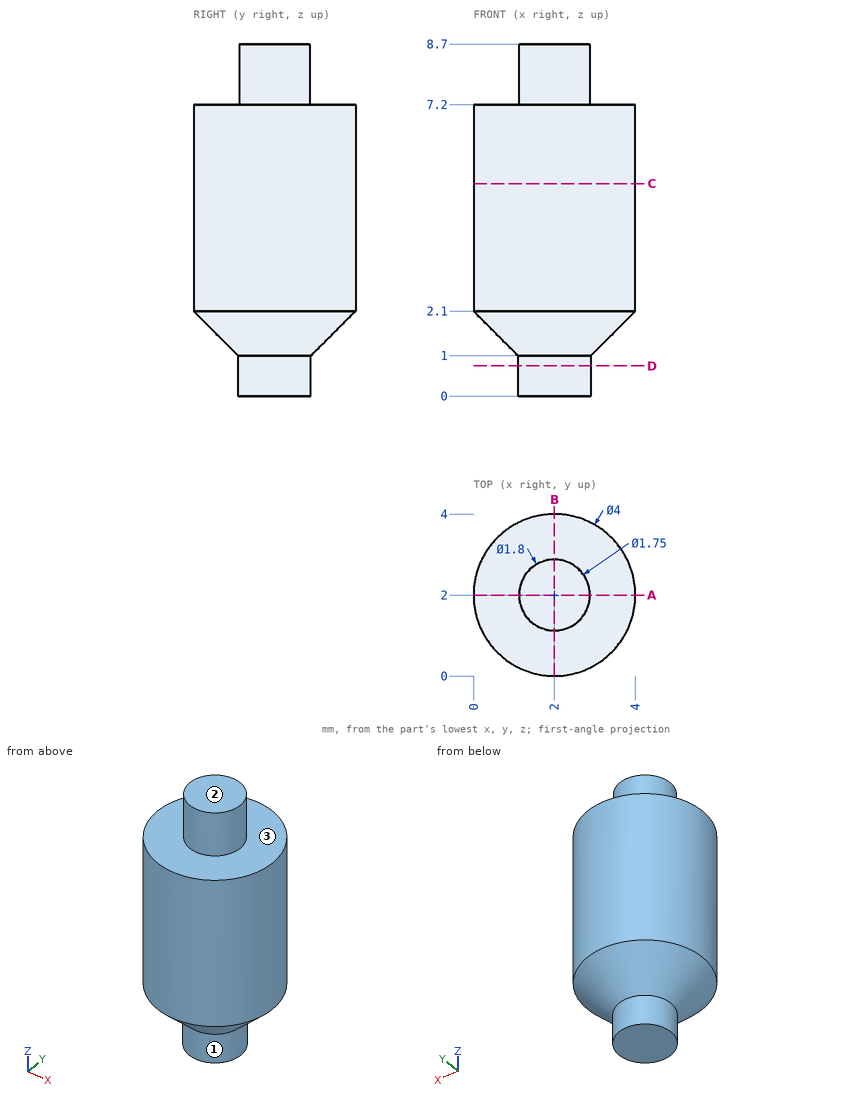
Here's the drawing with two shaded views (mm, measured from the low corner). I have some questions. A direction names the side the tool comes from. Give positions to 0.01 mm unless a question says otherwise; leave off trailing zeros. Loops run counter-clockwise (first coordinate to the right, second up) from the corner with the lowest first, then second, coordinate; pieces in that order, holes last. Notation, with made-up numbers: M 81.25,86.5 L 119.25,86.5 A15 ccw 119.25,113.5 Z; hole C 86,-17 d2. An arc over 180 degrees is marked long. One line per item, written item: value.
(1) Suppose I cut it at D-D on z = 0.75. List the corners of the cut face in (x, y) for me.
Returned:
outline: C 2,2 d1.8
(2) Will this pin go through, and if not, where does the flat tip stop? pin 1 (1.5 mm diameter, centred on x = 2, y = 3, fed in from +Z).
Returned:
pin 1: z = 8.7
(3) Suppose I cut it at C-C on z = 5.25. List the corners of the cut face in (x, y) for me.
Returned:
outline: C 2,2 d4
(4) Which directions (+Z, -Z, +X, -X, +Y, -Y) give clear straight access to the entire face, cutting with the end or side of a thin tool? Please do the marked faces 1, 2 and 3.
Returned:
face 1: -Z
face 2: +Z, +X, -X, +Y, -Y
face 3: +Z
(5) Suppose I cut it at A-A on y = 2. List the corners of the cut face in (x, z) for me (3 decimals).
Returned:
outline: M 0,2.1 L 1.1,1 L 1.1,0 L 2.9,0 L 2.9,1 L 4,2.1 L 4,7.2 L 2.875,7.2 L 2.875,8.7 L 1.125,8.7 L 1.125,7.2 L 0,7.2 Z
(6) I need wall thicknesses on line 1 (Z direction, x = 1.5, y = 2.9); line 2 (X direction, y = 3.5, z = 3.5); line 3 (Y direction, x = 2.6, z = 6.25). Which ranges of each line are inside material? Lowest first, please.
Returned:
line 1: 1.13 to 7.2
line 2: 0.68 to 3.32
line 3: 0.09 to 3.91
